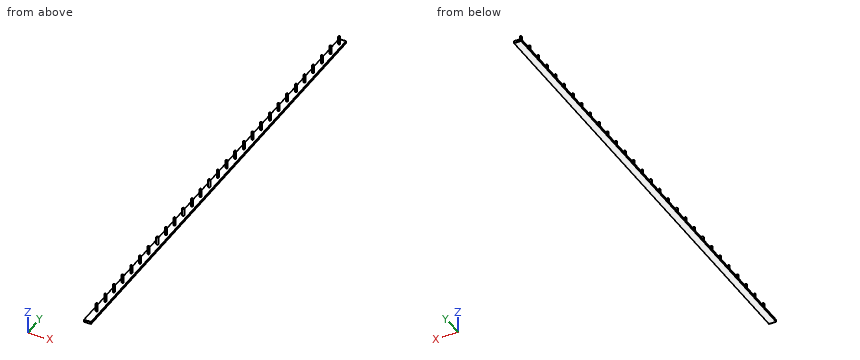
from build123d import *

# Parameters (mm, degrees)
SKETCH2_W           = 20.32
SKETCH2_H           = 1346.2
BOSS_EXTRUDE1_DEPTH = 6.35
SKETCH3_R           = 2.616420472
BOSS_EXTRUDE2_DEPTH = 22.86


with BuildPart() as part:
    # Sketch2 → Boss-Extrude1 (new body)
    with BuildSketch(Plane.XY):
        Rectangle(SKETCH2_W, SKETCH2_H)
    extrude(amount=BOSS_EXTRUDE1_DEPTH)

    # Sketch3 → Boss-Extrude2 (add)
    with BuildSketch(Plane.XY.offset(6.35)):
        with Locations((0.267312354, 654.853436839)):
            Circle(SKETCH3_R)
        with Locations((0.267312354, 609.133436839)):
            Circle(SKETCH3_R)
        with Locations((0.267312354, 563.413436839)):
            Circle(SKETCH3_R)
        with Locations((0.267312354, 517.693436839)):
            Circle(SKETCH3_R)
        with Locations((0.267312354, 471.973436839)):
            Circle(SKETCH3_R)
        with Locations((0.267312354, 426.253436839)):
            Circle(SKETCH3_R)
        with Locations((0.267312354, 380.533436839)):
            Circle(SKETCH3_R)
        with Locations((0.267312354, 334.813436839)):
            Circle(SKETCH3_R)
        with Locations((0.267312354, 289.093436839)):
            Circle(SKETCH3_R)
        with Locations((0.267312354, 243.373436839)):
            Circle(SKETCH3_R)
        with Locations((0.267312354, 197.653436839)):
            Circle(SKETCH3_R)
        with Locations((0.267312354, 151.933436839)):
            Circle(SKETCH3_R)
        with Locations((0.267312354, 106.213436839)):
            Circle(SKETCH3_R)
        with Locations((0.267312354, 60.493436839)):
            Circle(SKETCH3_R)
        with Locations((0.267312354, 14.773436839)):
            Circle(SKETCH3_R)
        with Locations((0.267312354, -30.946563161)):
            Circle(SKETCH3_R)
        with Locations((0.267312354, -76.666563161)):
            Circle(SKETCH3_R)
        with Locations((0.267312354, -122.386563161)):
            Circle(SKETCH3_R)
        with Locations((0.267312354, -168.106563161)):
            Circle(SKETCH3_R)
        with Locations((0.267312354, -213.826563161)):
            Circle(SKETCH3_R)
        with Locations((0.267312354, -259.546563161)):
            Circle(SKETCH3_R)
        with Locations((0.267312354, -305.266563161)):
            Circle(SKETCH3_R)
        with Locations((0.267312354, -350.986563161)):
            Circle(SKETCH3_R)
        with Locations((0.267312354, -396.706563161)):
            Circle(SKETCH3_R)
        with Locations((0.267312354, -442.426563161)):
            Circle(SKETCH3_R)
        with Locations((0.267312354, -488.146563161)):
            Circle(SKETCH3_R)
        with Locations((0.267312354, -533.866563161)):
            Circle(SKETCH3_R)
        with Locations((0.267312354, -579.586563161)):
            Circle(SKETCH3_R)
        with Locations((0.267312354, -625.306563161)):
            Circle(SKETCH3_R)
    extrude(amount=BOSS_EXTRUDE2_DEPTH)


solid = part.part
Build history of the part. All positions in model axes, mm. Round coordinates to 2 decimals unless told otherwise and drop trailing zeros. Write each loop counter-clockwise with the first axis right and the second up, starting at its lowest first coordinate (ties: lowest second). Pieces come first, ordered by that corner, then holes. Notation, with made-up numbers: M 32.25,-1.75 L 56.25,-1.75 A23 ccw 56.25,9.25 Z; hole C 40.25,-10 d3. An arc over 180 degrees is marked long. Answer in a Markdown table with one row per item.
1. Probe L1, parallel to Z at x = -3.75, y = 383.5; L2, parallel to X at y = 151, z = 19. List the from-to ranges inside material, lowest first. Write a range as [from, to].
Geometry check:
| item | result |
|---|---|
| L1 | [0, 6.35] |
| L2 | [-2.18, 2.71] |
2. Flat gauge pins, fed straight in: P1, Ø10, axis at y = 448.5, z = 11, coming from the -X side; P2, Ø4, axis at x = -3, y = -180, coming from the +Z side; P3, Ø3, axis at x = -1.5, z = 13.5, coming from the +Y side. Where does each tip first touch, or does it go through?
Geometry check:
| item | result |
|---|---|
| P1 | x = -10.16 |
| P2 | z = 6.35 |
| P3 | y = 657.46 |
3. Saw through at A-A (z = 23.5). State how many separate pieces and enclosed holes the cut face has, and give its area (3 significant figures).
Geometry check:
| item | result |
|---|---|
| separate pieces | 29 |
| enclosed holes | 0 |
| area | 624 mm2 |
4. Saw through at B-B (y = 366.5). List the corners of the cut face in (x, z).
Geometry check:
| item | result |
|---|---|
| outline | M -10.16,0 L 10.16,0 L 10.16,6.35 L -10.16,6.35 Z |
